Verification items for the finished model (mm, model axes). A direction names the side the tool comes from. Round coordinates to 2 decimals unless told otherwise and drop trailing zeros. Loops run counter-clockwise (first coordinate to the right, second up) from the corner with the lowest first, then second, coordinate; pieces in that order, holes last. Notation, with made-up numbers: (14, -22) -> (24, -22) arc R18 ccw to (24, 8) -> close; hole circle Ø5 at (-12, 89.25). An arc over 180 degrees is marked (long way). Write item = value, one per line.
```python
from build123d import *

# Parameters (mm, degrees)
SALIENTE_EXTRUIR1_DEPTH = 30
REDONDEO1_R             = 1


with BuildPart() as part:
    # Croquis1 → Saliente-Extruir1 (new body)
    with BuildSketch(Plane.XY):
        Polygon((-280, 180), (280, 180), (280, -180), (75, -180), (75, -150), (250, -150), (250, 150), (-250, 150), (-250, -150), (-75, -150), (-75, -180), (-280, -180), align=None)
    extrude(amount=SALIENTE_EXTRUIR1_DEPTH)

    # Redondeo1
    redondeo1_edges = [part.edges().sort_by_distance(p)[0] for p in [
        (177.5, -180, 30),
        (280, 0, 30),
        (0, 180, 30),
        (-280, 0, 30),
        (-177.5, -180, 30),
        (-75, -165, 30),
        (-162.5, -150, 30),
        (-250, 0, 30),
        (0, 150, 30),
        (250, 0, 30),
        (162.5, -150, 30),
        (75, -165, 30),
    ]]
    fillet(redondeo1_edges, radius=REDONDEO1_R)


solid = part.part
```
(1) Set-up check for faces 5 (the face through (-176, -180, 14)), 6 (the face through (75, -165, 14)), 7 (the face through (-250, 2, 14)): record each of +Z, -Z, +X, -X, +Y, -Y from which the full face is reachable in a straight line by a thin tool's end or side.
Filled sheet:
face_5 = +Z, -Z, +X, -X, -Y
face_6 = +Z, -Z, -Y
face_7 = +Z, -Z
(2) Sectioned sample at C-C, the plane z = 12. Record the cut outline in (x, y).
Filled sheet:
outline = (-280, -180) -> (-75, -180) -> (-75, -150) -> (-250, -150) -> (-250, 150) -> (250, 150) -> (250, -150) -> (75, -150) -> (75, -180) -> (280, -180) -> (280, 180) -> (-280, 180) -> close
(3) Sectioned sample at B-B, the plane x = 111.5. Record the cut outline in (y, z).
Filled sheet:
outline = (-180, 0) -> (-150, 0) -> (-150, 29) arc R1 ccw to (-151, 30) -> (-179, 30) arc R1 ccw to (-180, 29) -> close; (150, 0) -> (180, 0) -> (180, 29) arc R1 ccw to (179, 30) -> (151, 30) arc R1 ccw to (150, 29) -> close
(4) Go/stop test with a flat-tipped pin: pin 1 Ø10 at (x, z) = (15, 7) entering from -Y. Record where the tip stops, or that it passes through.
Filled sheet:
pin_1 = 150
(5) Material ranges on probe 1 along Y at (x, z) = (206, 23); probe 2 along X at (y, z) = (-41.5, 25.5); probe 3 along Y at (x, z) = (-38.5, 8.5), recorded low to high. Write a range as from..to.
Filled sheet:
probe_1 = -180..-150, 150..180
probe_2 = -280..-250, 250..280
probe_3 = 150..180
(6) Draft check along Y on faces 1 (the face through (250, -2, 14)), 2 (the face through (161, -150, 14)), 3 (the face through (280, 3, 14)), 4 (the face through (179, -180, 14)). Enter one of: released by +Y, released by -Y, zero draft, split by the parting line, or undercut.
Filled sheet:
face_1 = undercut
face_2 = undercut
face_3 = zero draft
face_4 = released by -Y
(7) Sectioned sample at A-A, the plane y = 58. Record the cut outline in (x, z), and give its area (3 significant figures).
Filled sheet:
outline = (-280, 0) -> (-250, 0) -> (-250, 29) arc R1 ccw to (-251, 30) -> (-279, 30) arc R1 ccw to (-280, 29) -> close; (250, 0) -> (280, 0) -> (280, 29) arc R1 ccw to (279, 30) -> (251, 30) arc R1 ccw to (250, 29) -> close
area = 1,800 mm2
(8) Sectioned sample at D-D, the plane x = 17. Record the cut outline in (y, z).
Filled sheet:
outline = (150, 0) -> (180, 0) -> (180, 29) arc R1 ccw to (179, 30) -> (151, 30) arc R1 ccw to (150, 29) -> close
